Autodesk Inventor part; units mm, degrees
ref_plane "YZ Plane" through (0, 0, 0) normal (1, 0, 0) x (0, 1, 0)
ref_plane "XZ Plane" through (0, 0, 0) normal (0, 1, 0) x (-1, 0, 0)
ref_plane "XY Plane" through (0, 0, 0) normal (0, 0, 1) x (1, 0, 0)
sketch "Sketch1" plane through (0, 0, 0) normal (1, 0, 0) x (0, 1, 0)
  line L0 (0, 0) -> (25.4, 0)
  line L1 (25.4, 0) -> (28.575, 0)
  line L2 (28.575, 0) -> (28.575, -12.7)
  line L3 (28.575, -12.7) -> (25.4, -12.7)
  line L4 (25.4, -12.7) -> (25.4, 0)
  line L5 (28.575, 0) -> (28.575, 31.75)
  line L6 (0, 0) -> (0, 6.35)
  line L7 (0, 6.35) -> (28.575, 31.75)
  line L8 (0, 0) -> (-3.175, 0)
  line L9 (-3.175, 0) -> (-3.175, -12.7)
  line L10 (-3.175, -12.7) -> (0, -12.7)
  line L11 (0, -12.7) -> (0, 0)
  line L12 (0, 6.35) -> (-3.175, 0)
  dimension "d0" = 25.4
  dimension "d1" = 3.175
  dimension "d2" = 12.7
  dimension "d3" = 31.75
  dimension "d16" = 6.35
  dimension "d17" = 3.175
extrude "Extrusion1" add sketch "Sketch1" along normal blind 53.34
sketch "Sketch2" plane through (0, 28.575, 31.75) normal (0, 1, 0) x (1, 0, 0)
  line L0 (53.34, 44.45) -> (53.34, 38.1)
  line L1 (53.34, 44.45) -> (53.34, 0)
  line L2 (53.34, 38.1) -> (26.67, 38.1)
  circle A0 centre (26.67, 38.1) radius 2.1082
  point P0 (0, 31.75)
  dimension "d6" = 6.35
  dimension "d7" = 26.67
  dimension "d8" = 4.2164
extrude "Extrusion2" cut sketch "Sketch2" against normal blind 43.815
sketch "Sketch3" plane through (53.34, 0, 0) normal (1, 0, 0) x (0, 0, -1)
  line L0 (12.7, 25.4) -> (12.7, 28.575)
  line L1 (12.7, 28.575) -> (-16.4619, 28.575)
  line L2 (-16.4619, 28.575) -> (-16.4619, 0)
  line L3 (-16.4619, 0) -> (12.7, 0)
  line L4 (12.7, 0) -> (12.7, 28.575)
  line L5 (-16.4619, 0) -> (-35.4962, 0)
  line L6 (-35.4962, 0) -> (-35.4962, 28.575)
  line L7 (-35.4962, 28.575) -> (-16.4619, 28.575)
  line L8 (-16.4619, 28.575) -> (-16.4619, 0)
  line L9 (12.7, -3.175) -> (12.7, 0)
  line L10 (12.7, 0) -> (-7.1998, 0)
  line L11 (-7.1998, 0) -> (-7.1998, -5.5168)
  line L12 (-7.1998, -5.5168) -> (12.7, -5.5168)
  line L13 (12.7, -5.5168) -> (12.7, 0)
  point P0 (0, 0)
  point P1 (12.7, 25.4)
extrude "Extrusion3" cut sketch "Sketch3" against normal blind 20.32
sketch "Sketch4" plane through (0, 28.575, 31.75) normal (0, 1, 0) x (1, 0, 0)
  circle A0 centre (26.67, 38.1) radius 2.1082
  line L0 (26.67, 38.1) -> (13.97, 38.1)
  circle A1 centre (13.97, 38.1) radius 2.1082
  point P0 (0, 31.75)
  dimension "d13" = 12.7
extrude "Extrusion4" cut sketch "Sketch4" against normal blind 2514.6 contours A1
fillet "Fillet1" radius 3.175 2 edges at (16.51, 0, 6.35) (16.51, -3.175, 0)
properties part number "sleds v2 big"
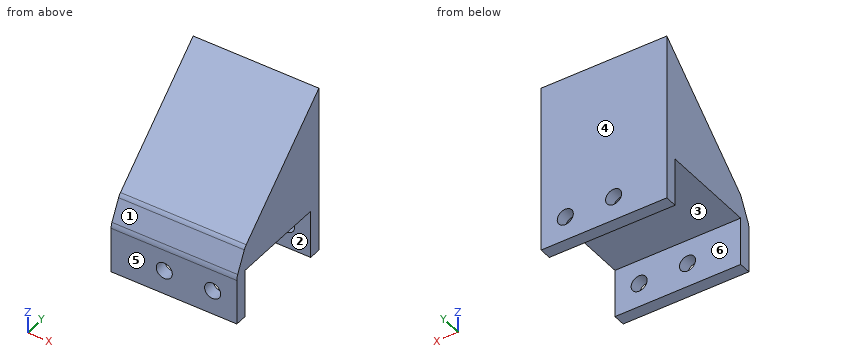
Source: CAD feature listing. Evaluate the final solid. Frame: model axes, mm. Face numbers are marked on the shaded views. A direction names the side the tool comes from. Give positions to 0.01 mm unless a question says otherwise; leave off trailing zeros. Write each loop counter-clockwise with the first axis right and the second up, starting at its lowest first coordinate (ties: lowest second). Pieces come first, ordered by that corner, then holes. Notation, with made-up numbers: M 79.5,64 L 121.5,64 A17 ccw 121.5,83 Z; hole C 87.5,72.5 d2. An arc over 180 degrees is marked long. Return JSON: item names as keys, results as strings. Group by question number.
1) Cut plane A-A, the plane x = 13.97. Output: boundary loops of the cut face in (y, z) (3 decimals).
2) Set-up query: the marked faces 1 and 2. Return all of +Z, -Z, +X, -X, +Y, -Y with unobstructed straight access to the full face (end or side cutting, diameter ignored); none if empty.
3) Material intervals for line 1 along X through (y, z) = (27.45, -6.35); line 2 along Y through (x, z) = (4.5, -9.5) (3 decimals); line 3 along Z through (x, y) = (13.97, -2.25), sorted ascending. Write a range as [from, to].
4) Pin query (flat end, axial travel): P1, Ø2, axis at x = 21, y = 16, coming from the +Z side; P2, Ø1, axis at x = 5, z = 1.5, coming from the -Y side (3 decimals); P3, Ø6, axis at x = 6.5, y = 20, coming from the -Z side. Return the tip coordinate at first contact, or that it passes through.
5) Pull-direction query (Y, two-part tool) for the marked faces 3, 4, 5 and 6; classes: pulls with the +Y half, pulls with the -Y half, needs draft (parallel to the pull), parting line crosses it, or undercut.
6) Cut plane C-C, the plane x = 20.5. Output: boundary loops of the cut face in (y, z) (3 decimals).
7) Cut plane B-B, the plane z = -6.35. Output: boundary loops of the cut face in (x, y) (3 decimals), plus the area to 3 significant figures.
8) Cut plane D-D, the plane x = 26. Output: boundary loops of the cut face in (y, z) (3 decimals), plus the area to 3 significant figures.
Recorded:
{
 "1": {"outline": "M -3.175,-12.7 L 0,-12.7 L 0,-8.458 L -3.175,-8.458 Z; M -3.175,-4.242 L 0,-4.242 L 0,0 L 25.4,0 L 25.4,-4.242 L 28.575,-4.242 L 28.575,31.75 L 0.457,6.756 A3.175 ccw -0.273,5.803 L -2.84,0.67 A3.175 ccw -3.175,-0.75 Z; M 25.4,-12.7 L 28.575,-12.7 L 28.575,-8.458 L 25.4,-8.458 Z"},
 "2": {"face 1": "+Z, +X, -X, -Y", "face 2": "-Z, +X, -X"},
 "3": {"line 1": "x = [0, 11.86], [16.08, 24.56], [28.78, 33.02]", "line 2": "y = [-3.175, 0], [25.4, 28.575]", "line 3": "z = [-12.7, -8.46], [-4.24, 1.85]"},
 "4": {"P1": "stops at z = 21.46", "P2": "stops at y = -2.675", "P3": "stops at z = 0"},
 "5": {"face 3": "undercut", "face 4": "pulls with the +Y half", "face 5": "pulls with the -Y half", "face 6": "undercut"},
 "6": {"outline": "M -3.175,-12.7 L 0,-12.7 L 0,0 L 25.4,0 L 25.4,-12.7 L 28.575,-12.7 L 28.575,31.75 L 0.457,6.756 A3.175 ccw -0.273,5.803 L -2.84,0.67 A3.175 ccw -3.175,-0.75 Z"},
 "7": {"outline": "M 0,-3.175 L 11.862,-3.175 L 11.862,0 L 0,0 Z; M 0,25.4 L 11.862,25.4 L 11.862,28.575 L 0,28.575 Z; M 16.078,-3.175 L 24.562,-3.175 L 24.562,0 L 16.078,0 Z; M 16.078,25.4 L 24.562,25.4 L 24.562,28.575 L 16.078,28.575 Z; M 28.778,-3.175 L 33.02,-3.175 L 33.02,0 L 28.778,0 Z; M 28.778,25.4 L 33.02,25.4 L 33.02,28.575 L 28.778,28.575 Z", "area": "156 mm²"},
 "8": {"outline": "M -3.175,-12.7 L 0,-12.7 L 0,-8.349 L -3.175,-8.349 Z; M -3.175,-4.351 L 0,-4.351 L 0,0 L 25.4,0 L 25.4,-4.351 L 28.575,-4.351 L 28.575,31.75 L 0.457,6.756 A3.175 ccw -0.273,5.803 L -2.84,0.67 A3.175 ccw -3.175,-0.75 Z; M 25.4,-12.7 L 28.575,-12.7 L 28.575,-8.349 L 25.4,-8.349 Z", "area": "610 mm²"}
}
